Geometry check sheet. Reference: the model listing, model coordinates, mm. Face numbers are marked on the shaded views. Give positions to 0.01 mm unless a question says otherwise; leave off trailing zeros. Write each loop counter-clockwise with the first axis right and the second up, starting at its lowest first coordinate (ties: lowest second). Pieces come first, ordered by that corner, then holes. Notation, with made-up numbers: M 24.25,74 L 45.25,74 A29 ccw 45.25,110 Z; hole C 16.25,87 d9. An arc over 180 degrees is marked long. One line per item, written item: value. Start each with the question number.
1. Cross-section at A-A on x = 7. Record the cut outline in (y, z).
2. Cross-section at B-B on x = 10.75. Record the cut outline in (y, z), then the cut area to 3 significant figures.
3. Scan lines: line 1 (Z direction, x = 5, y = 0); line 2 (Y direction, x = 1.3, z = 0); line 3 (Z direction, x = 2, y = 0). Record each from-to range of solid material in increasing order.
4. Release check for a two-part mould opening along Y. For the marked faces 1, 2 and 3 record: pulls with the +Y half, pulls with the -Y half, needs draft (parallel to the pull), parting line crosses it, or undercut.
5. Gauge pin test, flat ends, axial feed: pin 1 (3 mm diameter, centred on y = 23, z = 0, fed in from -X); pin 2 (2 mm diameter, centred on x = 15, z = 4, fed in from +Y); pin 3 (2 mm diameter, centred on x = 10, y = 15, fed in from -Z). Record the tip position at first contact, or that the pin passes through.
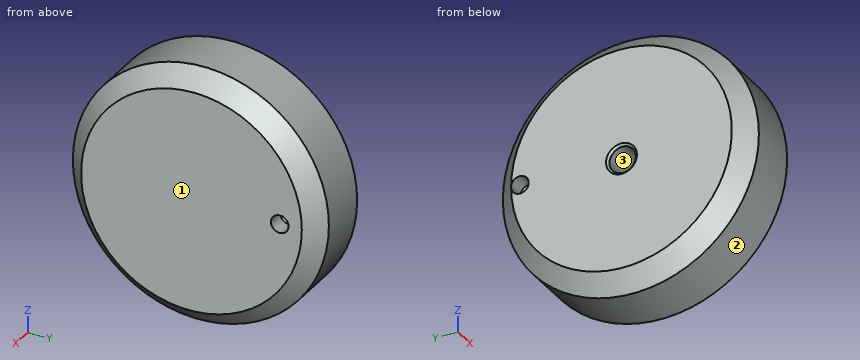
Autodesk Inventor part; units mm, degrees
ref_plane "YZ Plane" through (0, 0, 0) normal (1, 0, 0) x (0, 1, 0)
ref_plane "XZ Plane" through (0, 0, 0) normal (0, 1, 0) x (-1, 0, 0)
ref_plane "XY Plane" through (0, 0, 0) normal (0, 0, 1) x (1, 0, 0)
sketch "Эскиз5" plane through (0, 0, 0) normal (0, 0, 1) x (1, 0, 0)
  line L0 (0, 0) -> (20, 0)
  line L1 (20, 0) -> (20, 25)
  line L2 (16, 29) -> (4, 29)
  line L3 (0, 25) -> (0, 0)
  line L4 (4, 29) -> (0, 25)
  line L5 (16, 29) -> (20, 25)
  point P0 (20, 29)
  point P1 (0, 29)
  dimension "d42" = 20
  dimension "d43" = 29
  dimension "d44" = 4
  dimension "d45" = 4
  dimension "d46" = 4
  dimension "d47" = 4
revolve "Вращение3" add sketch "Эскиз5" angle 360 about axis through (0, 0, 0) along (1, 0, 0)
sketch "Эскиз6" plane through (0, 0, 0) normal (-1, 0, 0) x (0, 0, 1)
  point P0 (0, 0)
  point P1 (0, 0)
hole "Отверстие3" at (0, 0, 0) direction (1, 0, 0) diameter 6 depth 8 tip angle 140 countersink diameter 7 countersink angle 90
sketch "Эскиз8" plane through (0, 0, 0) normal (-1, 0, 0) x (0, 0, 1)
  line L0 (0, 0) -> (0, 23) construction
  dimension "d56" = 23
hole "Отверстие4" at (0, 23, 0) direction (1, 0, 0) diameter 4 depth 4
sketch "Эскиз9" plane through (20, 0, 0) normal (1, 0, 0) x (0, 0, -1)
  line L0 (0, 0) -> (0, 20) construction
  dimension "d64" = 20
hole "Отверстие5" at (20, 20, 0) direction (-1, 0, 0) diameter 4 depth 4 tip angle 118
thread "Резьба3"
properties part number "711138 (Доделать)"
Report:
1. outline: C 0,0 d58; hole C 0,0 d6
2. outline: C 0,0 d58
2. area: 2,640 mm^2
3. line 1: z = -29 to -3, 3 to 29
3. line 2: y = -26.3 to -3, 3 to 21, 25 to 26.3
3. line 3: z = -27 to -3, 3 to 27
4. face 1: needs draft
4. face 2: parting line crosses it
4. face 3: undercut
5. pin 1: stops at x = 4
5. pin 2: stops at y = 28.84
5. pin 3: stops at z = -25.4
